The listing builds one solid part. Answer for the finished solid, in the listing's coordinates (mm). Give positions to 0.01 mm unless a question says otherwise; leave off trailing zeros. Loops run counter-clockwise (first coordinate to the right, second up) from the corner with the lowest first, then second, coordinate; pieces in that order, holes last. Notation, with made-up numbers: M 29,-25.75 L 57,-25.75 A17 cw 57,6.25 Z; hole C -32.5,44 d1. An arc over 180 degrees is marked long. One line per item, written item: value. Start each with the question number.
Q1. Consider L1, parallel to Z at x = 91, y = 2.25; L2, parallel to X at y = 1.45, z = 0; L3, parallel to Z at x = -88, y = 2.3. Determine where each line is inside the solid, lowest interval first.
Q2. A cutting plane is placed at B-B, the plane z = -58. Determine the outline of the cut face in (x, y) (3 decimals), and give its area (3 significant figures).
Q3. A cutting plane is placed at D-D, the plane y = 2.15. State how many separate pieces and enclosed holes the cut face has, and give its area (3 significant figures).
Q4. A flat-ended cylindrical pin translates along its axis: pin 1 (20.5 mm diameter, centred on x = 90.551, z = 46.609, fed in from -Y). Find the tip coordinate at first contact, or state that the pin passes through.
Q5. A cutting plane is placed at A-A, the plane x = 152.4. Determine the outline of the cut face in (y, z) (3 decimals), and give its area (3 significant figures).
Q6. A cutting plane is placed at C-C, the plane x = -38.1. Determine the outline of the cut face in (y, z) (3 decimals).
from build123d import *

# Parameters (mm, degrees)
SKETCH1_W           = 330.2
SKETCH1_H           = 152.4
BOSS_EXTRUDE1_DEPTH = 3.175
SKETCH2_R           = 3.175
CUT_EXTRUDE1_DEPTH  = 4.175
SKETCH3_R           = 16.891
CUT_EXTRUDE2_DEPTH  = 4.175


with BuildPart() as part:
    # Sketch1 → Boss-Extrude1 (new body)
    with BuildSketch(Plane(origin=(0, 0, 0), x_dir=(1, 0, 0), z_dir=(0, 1, 0))):
        Rectangle(SKETCH1_W, SKETCH1_H)
    extrude(amount=BOSS_EXTRUDE1_DEPTH)

    # Sketch2 → Cut-Extrude1 (cut, through all)
    with BuildSketch(Plane(origin=(0, 3.175, 0), x_dir=(1, 0, 0), z_dir=(0, 1, 0))):
        with Locations((-152.4, 69.85)):
            Circle(SKETCH2_R)
        with Locations((-114.3, 69.85)):
            Circle(SKETCH2_R)
        with Locations((-76.2, 69.85)):
            Circle(SKETCH2_R)
        with Locations((-38.1, 69.85)):
            Circle(SKETCH2_R)
        with Locations((0, 69.85)):
            Circle(SKETCH2_R)
        with Locations((38.1, 69.85)):
            Circle(SKETCH2_R)
        with Locations((76.2, 69.85)):
            Circle(SKETCH2_R)
        with Locations((114.3, 69.85)):
            Circle(SKETCH2_R)
        with Locations((152.4, 69.85)):
            Circle(SKETCH2_R)
        with Locations((-114.3, -69.85)):
            Circle(SKETCH2_R)
        with Locations((-76.2, -69.85)):
            Circle(SKETCH2_R)
        with Locations((-38.1, -69.85)):
            Circle(SKETCH2_R)
        with Locations((0, -69.85)):
            Circle(SKETCH2_R)
        with Locations((38.1, -69.85)):
            Circle(SKETCH2_R)
        with Locations((76.2, -69.85)):
            Circle(SKETCH2_R)
        with Locations((114.3, -69.85)):
            Circle(SKETCH2_R)
        with Locations((152.4, -69.85)):
            Circle(SKETCH2_R)
        with Locations((-152.4, -69.85)):
            Circle(SKETCH2_R)
    extrude(amount=-CUT_EXTRUDE1_DEPTH, mode=Mode.SUBTRACT)

    # Sketch3 → Cut-Extrude2 (cut, through all)
    with BuildSketch(Plane(origin=(0, 3.175, 0), x_dir=(1, 0, 0), z_dir=(0, 1, 0))):
        with Locations((-122.809, 46.609)):
            Circle(SKETCH3_R)
        with Locations((-122.809, 0)):
            Circle(SKETCH3_R)
        with Locations((-122.809, -46.609)):
            Circle(SKETCH3_R)
        with Locations((-87.249, 23.3045)):
            Circle(SKETCH3_R)
        with Locations((-87.249, -23.3045)):
            Circle(SKETCH3_R)
        with Locations((-51.689, 0)):
            Circle(SKETCH3_R)
        with Locations((-51.689, -46.609)):
            Circle(SKETCH3_R)
        with Locations((-16.129, -23.3045)):
            Circle(SKETCH3_R)
        with Locations((-51.689, 46.609)):
            Circle(SKETCH3_R)
        with Locations((-16.129, 23.3045)):
            Circle(SKETCH3_R)
        with Locations((19.431, 0)):
            Circle(SKETCH3_R)
        with Locations((19.431, -46.609)):
            Circle(SKETCH3_R)
        with Locations((54.991, -23.3045)):
            Circle(SKETCH3_R)
        with Locations((19.431, 46.609)):
            Circle(SKETCH3_R)
        with Locations((54.991, 23.3045)):
            Circle(SKETCH3_R)
        with Locations((90.551, 0)):
            Circle(SKETCH3_R)
        with Locations((90.551, -46.609)):
            Circle(SKETCH3_R)
        with Locations((126.111, -23.3045)):
            Circle(SKETCH3_R)
        with Locations((90.551, 46.609)):
            Circle(SKETCH3_R)
        with Locations((126.111, 23.3045)):
            Circle(SKETCH3_R)
    extrude(amount=-CUT_EXTRUDE2_DEPTH, mode=Mode.SUBTRACT)


solid = part.part
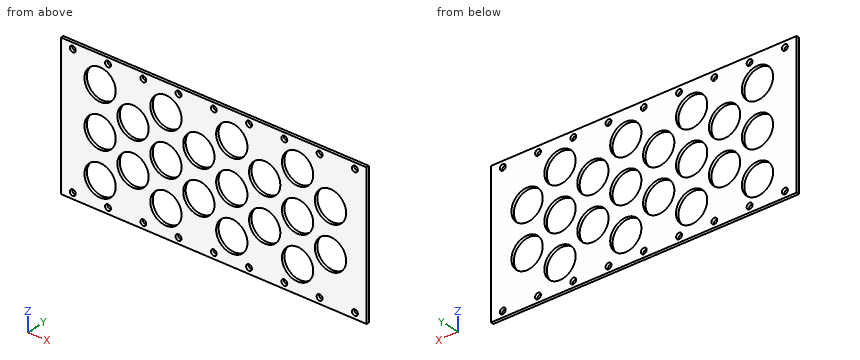
Answer block:
1. L1: -76.2 to -63.49, -29.72 to -16.89, 16.89 to 29.72, 63.49 to 76.2
1. L2: -165.1 to -139.7, -105.92 to -68.58, -34.8 to 2.54, 36.32 to 73.66, 107.44 to 165.1
1. L3: -76.2 to -40.18, -6.43 to 6.43, 40.18 to 76.2
2. outline: M -165.1,0 L -135.281,0 L -135.281,3.175 L -165.1,3.175 Z; M -110.337,0 L -64.161,0 L -64.161,3.175 L -110.337,3.175 Z; M -39.217,0 L 6.959,0 L 6.959,3.175 L -39.217,3.175 Z; M 31.903,0 L 78.079,0 L 78.079,3.175 L 31.903,3.175 Z; M 103.023,0 L 165.1,0 L 165.1,3.175 L 103.023,3.175 Z
2. area: 732 mm^2
3. separate pieces: 1
3. enclosed holes: 38
3. area: 31,800 mm^2
4. pin 1: through
5. outline: M 0,-76.2 L 3.175,-76.2 L 3.175,-73.025 L 0,-73.025 Z; M 0,-66.675 L 3.175,-66.675 L 3.175,66.675 L 0,66.675 Z; M 0,73.025 L 3.175,73.025 L 3.175,76.2 L 0,76.2 Z
5. area: 444 mm^2
6. outline: M 0,-76.2 L 3.175,-76.2 L 3.175,-73.025 L 0,-73.025 Z; M 0,-66.675 L 3.175,-66.675 L 3.175,-56.641 L 0,-56.641 Z; M 0,-36.577 L 3.175,-36.577 L 3.175,-10.032 L 0,-10.032 Z; M 0,10.032 L 3.175,10.032 L 3.175,36.577 L 0,36.577 Z; M 0,56.641 L 3.175,56.641 L 3.175,66.675 L 0,66.675 Z; M 0,73.025 L 3.175,73.025 L 3.175,76.2 L 0,76.2 Z
